Answer from the drawing. Dimensions are ordinates in mm from the lowest x, y and z of the part. Give positions to 0.01 mm unless a question says otherwise; leave off trailing zeros. Write each loop counter-clockwise with the first axis right and the second up, starting at its lowest first coordinate (ties: lowest second). Pieces come first, ordered by that corner, then holes.
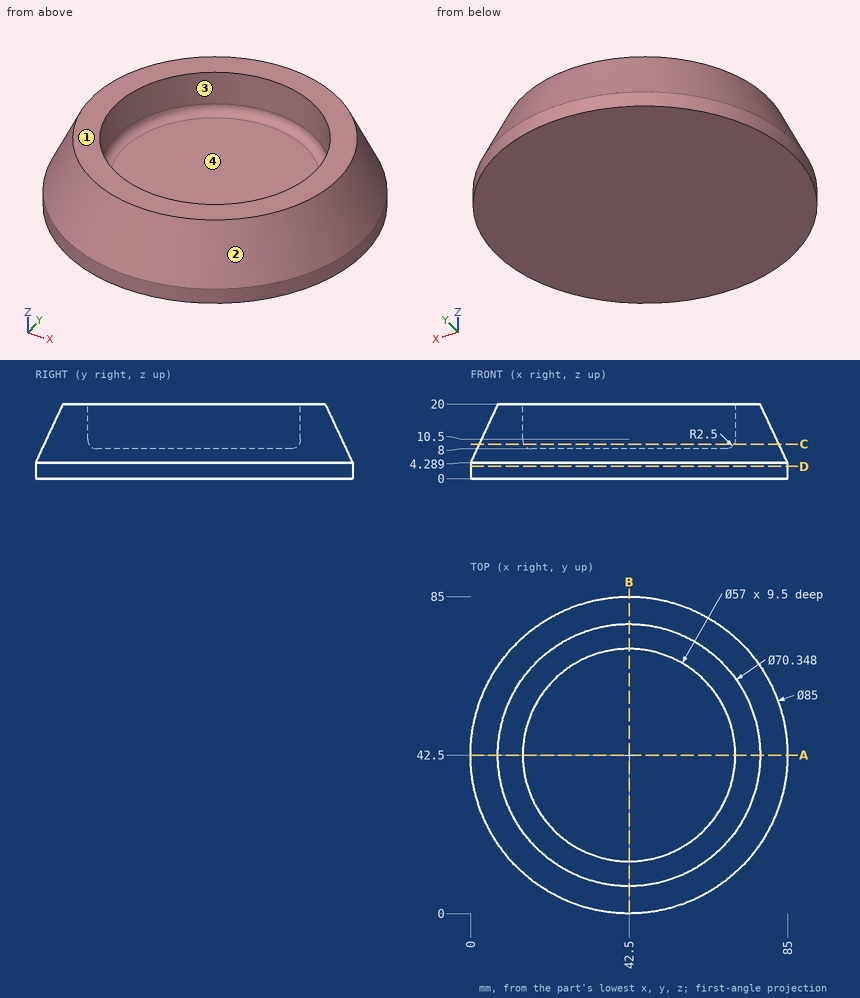
Item 1: Each of these flat-tipped pins is pushed along its axis until it touches: pin 1 Ø8 at (y, z) = (28.5, 6.5) entering from +X; pin 2 Ø2 at (x, z) = (43.5, 8) entering from -Y (1 decimal); pin 3 Ø2 at (y, z) = (76, 5.5) entering from +X (1 decimal). Where does it stop, or does it pass through?
Result set:
pin 1: stops at x = 83.64
pin 2: stops at y = 1.3
pin 3: stops at x = 69.2
Item 2: Determine the mould class of the marked faces 1, 2, 3 and 4 for opening direction X: pulls with the +X half, pulls with the -X half, needs draft (parallel to the pull), parting line crosses it, or undercut.
Result set:
face 1: needs draft
face 2: parting line crosses it
face 3: undercut
face 4: undercut
Item 3: Section C-C (z = 9.25) is taken. Write down the section's boundary in (x, y) (1 decimal), and give its area (3 significant figures).
Result set:
outline: circle Ø80.4 at (42.5, 42.5); hole circle Ø56.3 at (42.5, 42.5)
area: 2,580 mm2
Item 4: Section D-D (z = 3.25) is taken. Write down the section's boundary in (x, y), and give its area (3 significant figures).
Result set:
outline: circle Ø85 at (42.5, 42.5)
area: 5,670 mm2
Item 5: Section A-A (y = 42.5) is taken. Write down the section's boundary in (x, z).
Result set:
outline: (0, 0) - (85, 0) - (85, 4.29) - (77.67, 20) - (71, 20) - (71, 10.5) arc R2.5 cw to (68.5, 8) - (16.5, 8) arc R2.5 cw to (14, 10.5) - (14, 20) - (7.33, 20) - (0, 4.29) - close
Item 6: Find the intervals of material crossed by line 1 along Z through (x, y) = (52, 27.5); line 2 along Y through (x, z) = (42.5, 14); line 3 along Y through (x, z) = (65, 15.25) (1 decimal), in increasing order.
Result set:
line 1: z = 0 to 8
line 2: y = 4.53 to 14, 71 to 80.47
line 3: y = 12.6 to 25, 60 to 72.4
